```python
from build123d import *

# Parameters (mm, degrees)
F1_DEPTH = 3.556
F2_DEPTH = 12.192
F3_START = 12.192
F3_DEPTH = 2.9972


with BuildPart() as f1:
    # F0 (on Top) → F1 (new body)
    with BuildSketch(Plane.XY):
        Polygon((0, 25.4), (0, 0), (3.556, 0), (3.556, 21.844), (25.4, 21.844), (25.4, 25.4), align=None)
        with BuildLine():
            Line((3.556, 21.844), (3.556, 0))
            Line((3.556, 0), (6.731, 0))
            Line((6.731, 0), (6.731, 16.162614712))
            Line((6.731, 16.162614712), (5.5840602845, 17.3103928864))
            ThreePointArc((5.5840602845, 17.3103928864), (5.47330485, 17.412223604), (5.3715550967, 17.5230534241))
            ThreePointArc((5.3715550967, 17.5230534241), (5.3980463342, 19.8456556526), (7.6994134833, 20.1601268643))
            ThreePointArc((7.6994134833, 20.1601268643), (7.9854877449, 19.9289779751), (8.2178836864, 19.6439158442))
            Line((8.2178836864, 19.6439158442), (9.1970662222, 18.669))
            Line((9.1970662222, 18.669), (25.4, 18.669))
            Line((25.4, 18.669), (25.4, 21.844))
            Line((25.4, 21.844), (3.556, 21.844))
        make_face()
        with BuildLine():
            Line((6.731, 16.162614712), (6.731, 0))
            Line((6.731, 0), (19.05, 0))
            Line((19.05, 0), (19.05, 4.572))
            ThreePointArc((19.05, 4.572), (18.3692887661, 4.7074665251), (17.79230485, 5.093223604))
            Line((17.79230485, 5.093223604), (6.731, 16.162614712))
        make_face()
        with BuildLine():
            Line((19.05, 4.572), (19.05, 0))
            Line((19.05, 0), (25.4, 0))
            Line((25.4, 0), (25.4, 18.669))
            Line((25.4, 18.669), (9.1970662222, 18.669))
            Line((9.1970662222, 18.669), (20.3044877449, 7.6099779751))
            ThreePointArc((20.3044877449, 7.6099779751), (20.6919140067, 7.0322040712), (20.828, 6.35))
            ThreePointArc((20.828, 6.35), (20.3072358569, 5.0927641431), (19.05, 4.572))
        make_face()
    extrude(amount=F1_DEPTH)

    # F0 (on Top) → F2 (join)
    with BuildSketch(Plane.XY):
        Polygon((0, 25.4), (0, 0), (3.556, 0), (3.556, 21.844), (25.4, 21.844), (25.4, 25.4), align=None)
    extrude(amount=F2_DEPTH)

    # F0 (on Top) → F3 (join)
    with BuildSketch(Plane.XY.offset(F3_START)):
        with BuildLine():
            Line((3.556, 21.844), (3.556, 0))
            Line((3.556, 0), (6.731, 0))
            Line((6.731, 0), (6.731, 16.162614712))
            Line((6.731, 16.162614712), (5.5840602845, 17.3103928864))
            ThreePointArc((5.5840602845, 17.3103928864), (5.47330485, 17.412223604), (5.3715550967, 17.5230534241))
            ThreePointArc((5.3715550967, 17.5230534241), (5.3980463342, 19.8456556526), (7.6994134833, 20.1601268643))
            ThreePointArc((7.6994134833, 20.1601268643), (7.9854877449, 19.9289779751), (8.2178836864, 19.6439158442))
            Line((8.2178836864, 19.6439158442), (9.1970662222, 18.669))
            Line((9.1970662222, 18.669), (25.4, 18.669))
            Line((25.4, 18.669), (25.4, 21.844))
            Line((25.4, 21.844), (3.556, 21.844))
        make_face()
        with BuildLine():
            ThreePointArc((5.5840602845, 17.3103928864), (6.1203935178, 16.9991366152), (6.731, 16.891))
            Line((6.731, 16.891), (6.731, 18.669))
            Line((6.731, 18.669), (8.509, 18.669))
            ThreePointArc((8.509, 18.669), (8.4346671028, 19.1777262553), (8.2178836864, 19.6439158442))
            Line((8.2178836864, 19.6439158442), (7.6994134833, 20.1601268643))
            ThreePointArc((7.6994134833, 20.1601268643), (5.3980463342, 19.8456556526), (5.3715550967, 17.5230534241))
            Line((5.3715550967, 17.5230534241), (5.5840602845, 17.3103928864))
        make_face()
        with BuildLine():
            Line((5.5840602845, 17.3103928864), (6.731, 16.162614712))
            Line((6.731, 16.162614712), (6.731, 16.891))
            ThreePointArc((6.731, 16.891), (6.1203935178, 16.9991366152), (5.5840602845, 17.3103928864))
        make_face()
        with BuildLine():
            ThreePointArc((8.2178836864, 19.6439158442), (8.4346671028, 19.1777262553), (8.509, 18.669))
            Line((8.509, 18.669), (9.1970662222, 18.669))
            Line((9.1970662222, 18.669), (8.2178836864, 19.6439158442))
        make_face()
        Polygon((0, 25.4), (0, 0), (3.556, 0), (3.556, 21.844), (25.4, 21.844), (25.4, 25.4), align=None)
    extrude(amount=F3_DEPTH)


solid = f1.part
```
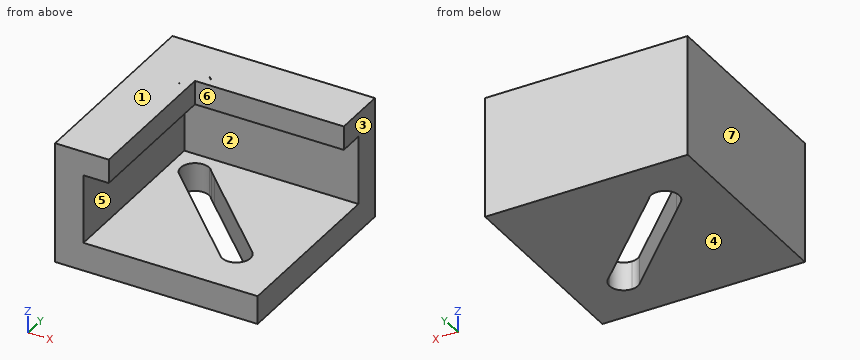
Can you work these out from the model? Positions are in its coordinate system, mm. Face numbers are marked on the shaded views. A direction names the side the tool comes from. Coordinates: 2 decimals unless noted, no trailing zeros. Loops run counter-clockwise (first coordinate to the right, second up) from the corner with the lowest first, then second, coordinate; pieces in that order, holes last.
1) Which directions (+Z, -Z, +X, -X, +Y, -Y) give clear straight access to the entire face, cutting with the end or side of a thin tool? Please do the marked faces 5, 6 and 7.
2) Imagine slicing it at A-A on z = 13.25. List the corners of the cut face in (x, y) for me.
3) For pin 1 (6.5 mm diameter, centred on x = 18, y = 11.5, fed in from +Z); pin 2 (4.5 mm diameter, centred on x = 16.5, z = 9, fed in from -Y); pin 3 (2 mm diameter, centred on y = 12.5, z = 7.5, fed in from +X), each with a flat end and sliding along its axis, tell me the tip position at first contact or that it passes through.
4) Imagine slicing it at B-B on y = 15.5. List the corners of the cut face in (x, z) for me, plus the area to 3 significant figures.
5) Imagine slicing it at D-D on z = 4.5. List the corners of the cut face in (x, y) for me.
6) Imagine slicing it at C-C on x = 15.5. List the corners of the cut face in (y, z) for me.
7) Thinking about a two-plate mould opening in Z: for the marked faces 1, 2, 3 and 4, which applies, pulls with the +Z half, pulls with the -Z half, needs draft (parallel to the pull), parting line crosses it, or undercut?
8) I need wall thicknesses on probe 1 along Z at (x, y) = (6, 13.25); probe 2 along Y at (x, z) = (10, 12); probe 3 along Z at (x, y) = (22, 18). Which ranges of each line are inside material? Lowest first, please.
Completed:
1. face 5: +X, -Y
1. face 6: +Z, +X, -Y
1. face 7: +Z, -Z, -X, +Y, -Y
2. outline: (0, 0) - (6.73, 0) - (6.73, 18.67) - (25.4, 18.67) - (25.4, 25.4) - (0, 25.4) - close; hole (5.37, 17.52) arc R1.78 ccw to (5.58, 17.31) - close; hole (7.7, 20.16) - (8.22, 19.64) arc R1.78 ccw to start
3. pin 1: stops at z = 3.56
3. pin 2: stops at y = 21.84
3. pin 3: stops at x = 3.56
4. outline: (0, 0) - (7.39, 0) - (7.39, 3.56) - (3.56, 3.56) - (3.56, 12.19) - (6.73, 12.19) - (6.73, 15.19) - (0, 15.19) - close; (12.38, 0) - (25.4, 0) - (25.4, 3.56) - (12.38, 3.56) - close
4. area: 123 mm2
5. outline: (0, 0) - (3.56, 0) - (3.56, 21.84) - (25.4, 21.84) - (25.4, 25.4) - (0, 25.4) - close
6. outline: (0, 0) - (7.39, 0) - (7.39, 3.56) - (0, 3.56) - close; (12.39, 0) - (25.4, 0) - (25.4, 15.19) - (18.67, 15.19) - (18.67, 12.19) - (21.84, 12.19) - (21.84, 3.56) - (12.39, 3.56) - close
7. face 1: pulls with the +Z half
7. face 2: undercut
7. face 3: needs draft
7. face 4: pulls with the -Z half
8. probe 1: z = 0 to 3.56, 12.19 to 15.19
8. probe 2: y = 21.84 to 25.4
8. probe 3: z = 0 to 3.56
